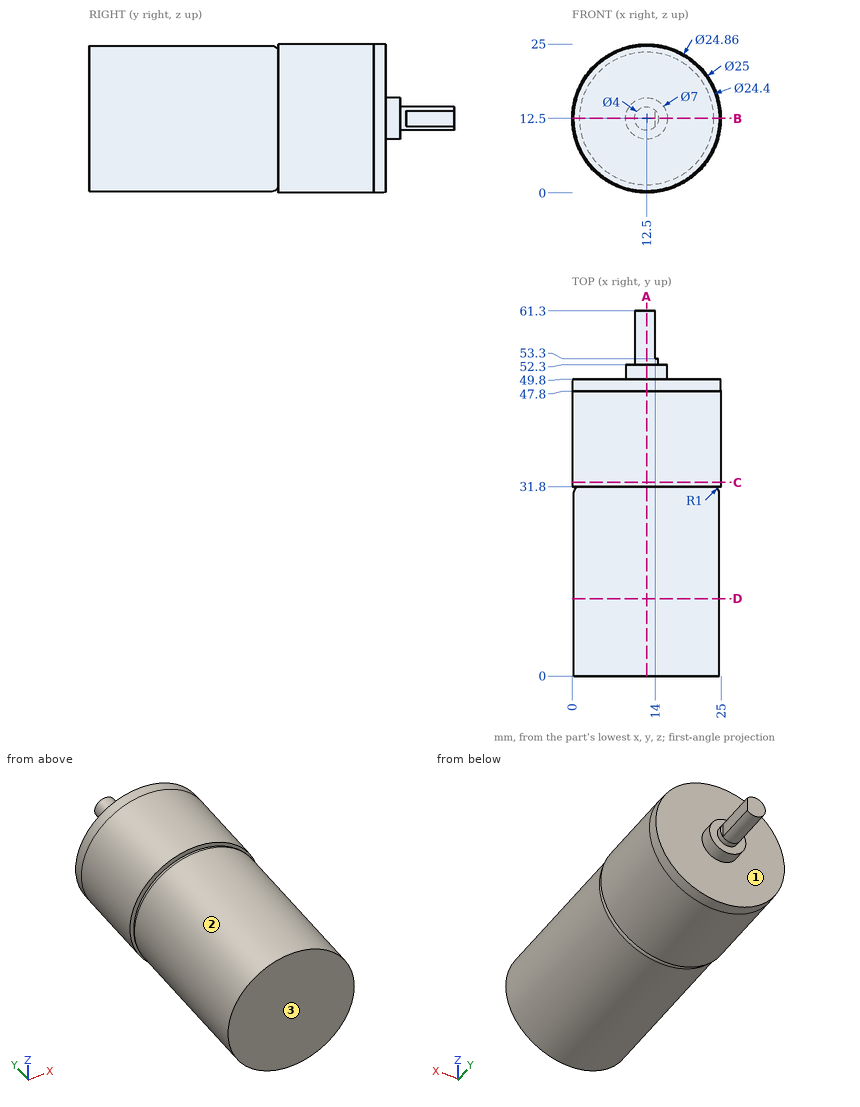
Drawing for the job (mm, zero at the part's lowest x, y, z). A direction names the side the tool comes from. Round coordinates to 2 decimals unless told otherwise and drop trailing zeros. Order: outer loops, then holes, each group sorted by start corner. A loop starts at its lowest first (then second) coordinate and runs counter-clockwise, first axis right, second up.
Item 1: Probe line 1 along Y through (x, z) = (18.5, 7); line 2 along X through (y, z) = (49.5, 12); line 3 along Z through (x, y) = (12.25, 9). List the from-to ranges inside material, lowest first.
Item 2: Saw through at A-A on x = 12.5. Write the cut outline in (y, z).
Item 3: Saw through at B-B on z = 12.5. Write the cut outline in (x, y), then the cut area to 3 significant figures.
Item 4: Saw through at C-C on y = 32.5. Write the cut outline in (x, z), then the cut area to 3 significant figures.
Item 5: Tool access for the marked faces 1, 2 and 3: list every direction of +Z, -Z, +X, -X, +Y, -Y with a clear straight run to the whole face (end or side of a thin tool).
Item 6: Pin check, flat tips, straight feed: pin 1 (12 mm diameter, centred on x = 19, y = 36, fed in from -Z); pin 2 (6 mm diameter, centred on x = 2.5, y = 25.5, fed in from +Z); pin 3 (1.5 mm diameter, centred on x = 21.5, z = 16, fed in from +Y). Stop position of each tip, or through.
Item 7: Saw through at D-D on y = 13. Write the cut outline in (x, z), then the cut area to 3 significant figures.
Reported:
1. line 1: y = 0 to 49.8
1. line 2: x = 0.07 to 24.93
1. line 3: z = 0.3 to 24.7
2. outline: (0, 0.3) - (30.8, 0.3) arc R1 ccw to (31.8, 1.3) - (31.8, 0) - (47.8, 0) - (49.8, 0.07) - (49.8, 9) - (52.3, 9) - (52.3, 10.5) - (61.3, 10.5) - (61.3, 14.5) - (52.3, 14.5) - (52.3, 16) - (49.8, 16) - (49.8, 24.93) - (47.8, 25) - (31.8, 25) - (31.8, 23.7) arc R1 ccw to (30.8, 24.7) - (0, 24.7) - close
3. outline: (0, 31.8) - (1.3, 31.8) arc R1 ccw to (0.3, 30.8) - (0.3, 0) - (24.7, 0) - (24.7, 30.8) arc R1 ccw to (23.7, 31.8) - (25, 31.8) - (25, 47.8) - (24.93, 49.8) - (16, 49.8) - (16, 52.3) - (14.5, 52.3) - (14.5, 53.3) - (14, 53.3) - (14, 61.3) - (10.5, 61.3) - (10.5, 52.3) - (9, 52.3) - (9, 49.8) - (0.07, 49.8) - (0, 47.8) - close
3. area: 1,270 mm2
4. outline: circle Ø25 at (12.5, 12.5)
4. area: 491 mm2
5. face 1: +Y
5. face 2: -Y
5. face 3: +Z, -Z, +X, -X, -Y
6. pin 1: stops at z = 0.01
6. pin 2: stops at z = 22.49
6. pin 3: stops at y = 49.8
7. outline: circle Ø24.4 at (12.5, 12.5)
7. area: 468 mm2
